from build123d import *

# Parameters (mm, degrees)
BOSS_EXTRUDE1_DEPTH = 153
SKETCH2_R           = 12
CUT_EXTRUDE1_DEPTH  = 213
SKETCH3_R           = 1.5
CUT_EXTRUDE2_DEPTH  = 10


with BuildPart() as part:
    # Sketch1 → Boss-Extrude1 (new body)
    with BuildSketch(Plane.XY):
        Polygon((0, -13.289354466), (-22.2, -13.289354466), (-22.2, -14.545627613), (-16.612166923, -23.689354466), (-16.612166923, -27.689354466), (-18.855505392, -27.689354466), (-26.2, -15.671090562), (-26.2, -9.289354466), (26.2, -9.289354466), (26.2, -15.671090562), (18.855505392, -27.689354466), (16.612166923, -27.689354466), (16.612166923, -23.689354466), (22.2, -14.545627613), (22.2, -13.289354466), align=None)
    extrude(amount=BOSS_EXTRUDE1_DEPTH)

    # Sketch2 → Cut-Extrude1 (cut)
    with BuildSketch(Plane(origin=(0, -9.289354466, 0), x_dir=(1, 0, 0), z_dir=(0, 1, 0))):
        with Locations(Location((0, -31.5, 0), (0, 0, 180))):
            Circle(SKETCH2_R)
        with Locations(Location((0, -76.5, 0), (0, 0, 180))):
            Circle(SKETCH2_R)
        with Locations(Location((0, -121.5, 0), (0, 0, 180))):
            Circle(SKETCH2_R)
    extrude(amount=-CUT_EXTRUDE1_DEPTH, mode=Mode.SUBTRACT)

    # Sketch3 → Cut-Extrude2 (cut)
    with BuildSketch(Plane(origin=(0, -9.289354466, 0), x_dir=(1, 0, 0), z_dir=(0, 1, 0))):
        with Locations(Location((-10, -99, 0), (0, 0, 180))):
            Circle(SKETCH3_R)
        with Locations((10, -99)):
            Circle(SKETCH3_R)
        with Locations(Location((10, -54, 0), (0, 0, 180))):
            Circle(SKETCH3_R)
        with Locations((-10, -54)):
            Circle(SKETCH3_R)
    extrude(amount=-CUT_EXTRUDE2_DEPTH, mode=Mode.SUBTRACT)


solid = part.part
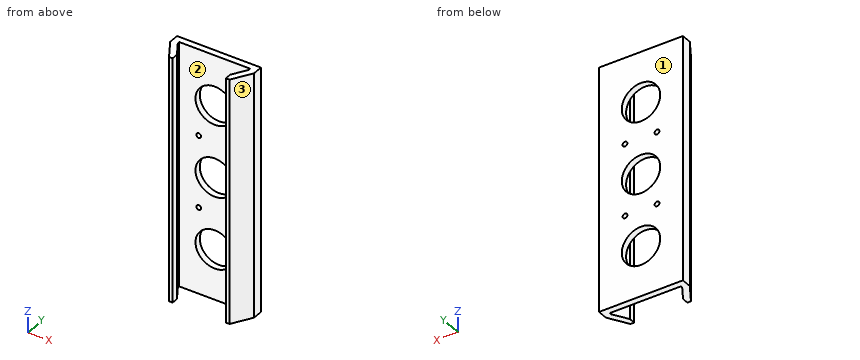
Geometry: final body of the model. Coordinates: model frame, mm. Face numbers are marked on the shaded views. Round coordinates to 2 decimals unless told otherwise and drop trailing zeros. Loops run counter-clockwise (first coordinate to the right, second up) from the corner with the lowest first, then second, coordinate; pieces in that order, holes last.
Q1. Material intervals for L1, parallel to Z at x = 0, y = -12.1; L2, parallel to X at y = -11.95, z = 99; L3, parallel to X at y = -13.5, z = 30, sorted ascending.
Q2. Pin query (flat end, axial travel): P1, Ø1.2, axis at y = -26, z = 56.5, coming from the -X side; P2, Ø1.2, axis at y = -24.5, z = 39, coming from the +X side; P3, Ø3.5, axis at x = -10, z = 54, coming from the -Y side; P4, Ø4, axis at x = 10, z = 54, coming from the +Y side. Return the tip coordinate at first contact, or that it passes through.
Q3. Section C-C on x = 0. Return loops of the section in (y, z).
Q4. Section B-B on y = -11.5. Return loops of the section in (x, z).
Q5. Pull-direction query (X, two-part tool) for the marked faces 1, 2 and 3; classes: released by +X, released by -X, zero draft, split by the parting line, or undercut.
Q6. Section D-D on z = 99. Return loops of the section in (x, y).
Q7. Section A-A on z = 76.5. Return loops of the section in (x, y), plus the area to 3 significant figures.
Evaluation:
1. L1: z = 0 to 19.5, 43.5 to 64.5, 88.5 to 109.5, 133.5 to 153
1. L2: x = -26.2 to -11.5, -8.5 to 8.5, 11.5 to 26.2
1. L3: x = -26.2 to -22.2, 22.2 to 26.2
2. P1: stops at x = -20.25
2. P2: stops at x = 21.17
2. P3: stops at y = -13.29
2. P4: stops at y = -9.29
3. outline: (-13.29, 0) - (-9.29, 0) - (-9.29, 19.5) - (-13.29, 19.5) - close; (-13.29, 43.5) - (-9.29, 43.5) - (-9.29, 64.5) - (-13.29, 64.5) - close; (-13.29, 88.5) - (-9.29, 88.5) - (-9.29, 109.5) - (-13.29, 109.5) - close; (-13.29, 133.5) - (-9.29, 133.5) - (-9.29, 153) - (-13.29, 153) - close
4. outline: (-26.2, 0) - (26.2, 0) - (26.2, 153) - (-26.2, 153) - close; hole circle Ø24 at (0, 31.5); hole circle Ø24 at (0, 76.5); hole circle Ø24 at (0, 121.5); hole circle Ø3 at (-10, 54); hole circle Ø3 at (-10, 99); hole circle Ø3 at (10, 54); hole circle Ø3 at (10, 99)
5. face 1: zero draft
5. face 2: undercut
5. face 3: released by +X
6. outline: (-26.2, -15.67) - (-18.86, -27.69) - (-16.61, -27.69) - (-16.61, -23.69) - (-22.2, -14.55) - (-22.2, -13.29) - (-11.5, -13.29) - (-11.5, -9.29) - (-26.2, -9.29) - close; (-8.5, -13.29) - (8.5, -13.29) - (8.5, -9.29) - (-8.5, -9.29) - close; (11.5, -13.29) - (22.2, -13.29) - (22.2, -14.55) - (16.61, -23.69) - (16.61, -27.69) - (18.86, -27.69) - (26.2, -15.67) - (26.2, -9.29) - (11.5, -9.29) - close
7. outline: (-26.2, -15.67) - (-18.86, -27.69) - (-16.61, -27.69) - (-16.61, -23.69) - (-22.2, -14.55) - (-22.2, -13.29) - (-12, -13.29) - (-12, -9.29) - (-26.2, -9.29) - close; (12, -13.29) - (22.2, -13.29) - (22.2, -14.55) - (16.61, -23.69) - (16.61, -27.69) - (18.86, -27.69) - (26.2, -15.67) - (26.2, -9.29) - (12, -9.29) - close
7. area: 236 mm2
